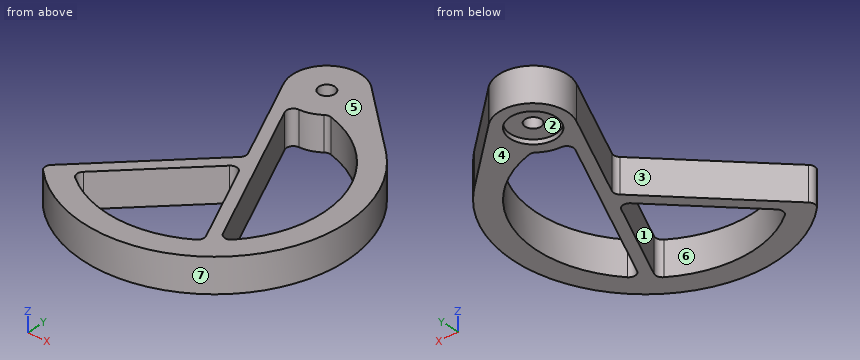
```python
from build123d import *

# Parameters (mm, degrees)
EXTRUDE_1_DEPTH     = 15
SKETCH_6_R          = 3.5
CUT_EXTRUDE_2_DEPTH = 15
SKETCH_8_R          = 10.1
CUT_EXTRUDE_4_DEPTH = 2


with BuildPart() as part:
    # ｽｹｯﾁ1 → ﾎﾞｽ - 押し出し1 (new body)
    with BuildSketch(Plane.XY):
        with BuildLine():
            Line((10.546944731, 68.165925034), (9.641814145, 68.990666647))
            ThreePointArc((9.641814145, 68.990666647), (-9.131421435, 69.400300104), (-13.594616806, 51.160726074))
            Line((-13.594616806, 51.160726074), (4.986432096, 11.313538113))
            ThreePointArc((4.986432096, 11.313538113), (5.221931994, 9.524738795), (4.388829079, 7.924362985))
            Line((4.388829079, 7.924362985), (-40.303464689, -36.767930783))
            ThreePointArc((-40.303464689, -36.767930783), (-41.182112782, -38.903012739), (-40.283913759, -41.029943849))
            ThreePointArc((-40.283913759, -41.029943849), (41.397896806, -39.905690573), (39.524106652, 41.762363359))
            Line((39.524106652, 41.762363359), (37.916838192, 43.226882625))
            Line((37.916838192, 43.226882625), (10.546944731, 68.165925034))
        make_face()
        with BuildLine():
            ThreePointArc((5.093338956, 1.55780505), (7.735603832, 2.390907965), (9.933582661, 0.704339492))
            Line((9.933582661, 0.704339492), (27.046217634, -35.993824637))
            ThreePointArc((27.046217634, -35.993824637), (27.212084573, -38.085077821), (25.967336583, -39.773702754))
            ThreePointArc((25.967336583, -39.773702754), (-1.972837213, -47.459012983), (-29.17877254, -37.481318454))
            ThreePointArc((-29.17877254, -37.481318454), (-30.330146685, -35.299826939), (-29.457223039, -32.992756945))
            Line((-29.457223039, -32.992756945), (5.093338956, 1.55780505))
        make_face(mode=Mode.SUBTRACT)
        with BuildLine():
            ThreePointArc((35.231836325, -31.858557864), (32.560090836, -32.813013733), (30.287744354, -31.114293205))
            Line((30.287744354, -31.114293205), (-2.054746852, 38.244403012))
            ThreePointArc((-2.054746852, 38.244403012), (-1.895310582, 41.077194163), (0.553480425, 42.510214831))
            ThreePointArc((0.553480425, 42.510214831), (5.039223996, 43.371793408), (9.057681155, 45.543478261))
            ThreePointArc((9.057681155, 45.543478261), (10.270904088, 46.091905397), (11.601973614, 46.061309233))
            ThreePointArc((11.601973614, 46.061309233), (45.455779175, 13.784851815), (35.231836325, -31.858557864))
        make_face(mode=Mode.SUBTRACT)
    extrude(amount=EXTRUDE_1_DEPTH)

    # ｽｹｯﾁ6 → ｶｯﾄ - 押し出し2 (cut)
    with BuildSketch(Plane.XY.offset(15)):
        with Locations((0, 57.5)):
            Circle(SKETCH_6_R)
    extrude(amount=-CUT_EXTRUDE_2_DEPTH, mode=Mode.SUBTRACT)

    # ｽｹｯﾁ8 → ｶｯﾄ - 押し出し4 (cut)
    with BuildSketch(Plane(origin=(0, 0, 0), x_dir=(-1, 0, 0), z_dir=(0, 0, -1))):
        with Locations((0, 57.5)):
            Circle(SKETCH_8_R)
    extrude(amount=-CUT_EXTRUDE_4_DEPTH, mode=Mode.SUBTRACT)


solid = part.part
```
Could you check a few things on this model? Use its own coordinates, in mm. Face numbers are marked on the shaded views. A direction names the side the tool comes from. Round coordinates to 2 decimals unless told otherwise and drop trailing zeros. Loops run counter-clockwise (first coordinate to the right, second up) from the corner with the lowest first, then second, coordinate; pieces in that order, holes last. Notation, with made-up numbers: (32, -33) -> (50, -33) arc R30 ccw to (50, -9) -> close; hole circle Ø2 at (66, -22.5). An arc over 180 degrees is marked (long way). Put each result on its own line as item: value.
Q1. For pin 1 Ø1 at (y, z) = (-28, 7.5) entering from -X; pin 2 Ø2 at (x, z) = (4.5, 6) entering from +Y; pin 3 Ø1.5 at (y, z) = (-4, 3) entering from +X, each with a flat end and sliding along its axis, tell me the tip position at first contact or that it passes through.
Checks:
pin 1: x = -32.04
pin 2: y = 72.09
pin 3: x = 57.41
Q2. Which directions (+Z, -Z, +X, -X, +Y, -Y) give clear straight access to the entire face, cutting with the end or side of a thin tool? Please do the marked faces 1, 2, 3 and 4.
Checks:
face 1: +Z, -Z
face 2: -Z
face 3: +Z, -Z, -X
face 4: -Z, +X, -X, +Y, -Y
Q3. I want a section at C-C on x = -5.5. Write out the boundary of the cut face in (y, z).
Checks:
outline: (-57.24, 0) -> (-47.18, 0) -> (-47.18, 15) -> (-57.24, 15) -> close; (-9.04, 0) -> (-1.96, 0) -> (-1.96, 15) -> (-9.04, 15) -> close; (33.8, 0) -> (49.03, 0) -> (49.03, 2) -> (65.97, 2) -> (65.97, 0) -> (71.46, 0) -> (71.46, 15) -> (33.8, 15) -> close
Q4. I want a section at B-B on y = 57.5. Write out the boundary of the cut face in (x, z).
Checks:
outline: (-15, 0) -> (-10.1, 0) -> (-10.1, 2) -> (-3.5, 2) -> (-3.5, 15) -> (-15, 15) -> close; (3.5, 2) -> (10.1, 2) -> (10.1, 0) -> (22.25, 0) -> (22.25, 15) -> (3.5, 15) -> close
Q5. Please list where these lines run through material, in increasing order: line 1 (Y direction, x = 0, z = 0.55); line 2 (Y direction, x = 0, z = 9.25); line 3 (Y direction, x = 16.5, z = 4). Write a range as from..to.
Checks:
line 1: -57.5..-47.5, -3.54..3.54, 22.01..33.84, 42.44..47.4, 67.6..72.5
line 2: -57.5..-47.5, -3.54..3.54, 22.01..33.84, 42.44..54, 61..72.5
line 3: -55.08..-44.54, -13.38..-1.55, 44.54..62.74
Q6. Thinking about a two-plate mould opening in Y: for the marked faces 5, 6 and 7, which applies, pulls with the +Y half, pulls with the -Y half, needs draft (parallel to the pull), parting line crosses it, or undercut?
Checks:
face 5: needs draft
face 6: undercut
face 7: parting line crosses it
